Design review of the part built by this model. Coordinates are the model's own, in mm. Face numbers are marked on the shaded views. A direction names the side the tool comes from. Round coordinates to 2 decimals unless told otherwise and drop trailing zeros. Write each loop counter-clockwise with the first axis right and the second up, starting at its lowest first coordinate (ties: lowest second). Pieces come first, ordered by that corner, then holes. Notation, with made-up numbers: M 3,49.25 L 46,49.25 A36 ccw 46,83.25 Z; hole C -37,11.5 d4. An arc over 180 degrees is marked long. Use CSV: the item, a comma, the result in double quotes.
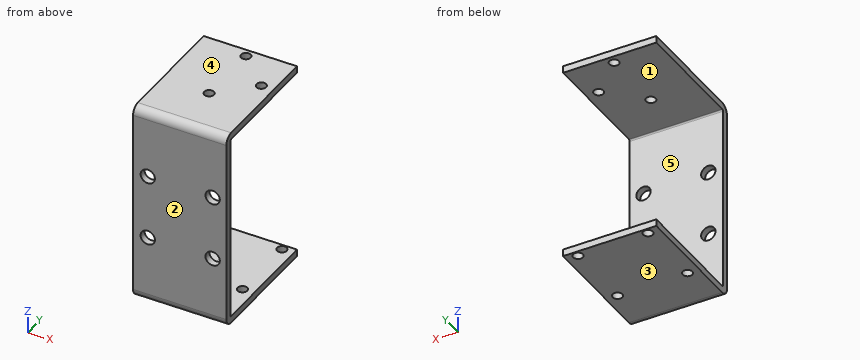
Autodesk Inventor part; units mm, degrees
ref_plane "YZ Plane" through (0, 0, 0) normal (1, 0, 0) x (0, 1, 0)
ref_plane "XZ Plane" through (0, 0, 0) normal (0, 1, 0) x (-1, 0, 0)
ref_plane "XY Plane" through (0, 0, 0) normal (0, 0, 1) x (1, 0, 0)
sketch "Sketch1" plane through (0, 0, 0) normal (0, 1, 0) x (-1, 0, 0)
  line L0 (10.17, 20.25) -> (-9.97, 20.25)
  line L1 (-9.97, 20.25) -> (-9.97, -20.25)
  line L2 (-9.97, -20.25) -> (10.17, -20.25)
  line L3 (10.17, -20.25) -> (10.17, 20.25)
  point P0 (0, 0)
  dimension "d0" = 40.5
  dimension "d1" = 20.14
  dimension "d2" = 10.17
  dimension "d3" = 20.25
extrude "Plate1" add sketch "Sketch1" along normal blind 1.5
sketch "Sketch2" plane through (9.97, 0, 21.75) normal (0, 0, -1) x (-1, 0, 0)
  line L0 (20.14, 0) -> (0, 0)
  line L1 (0, 0) -> (0, 26.9)
  line L2 (0, 26.9) -> (20.14, 26.9)
  line L3 (20.14, 26.9) -> (20.14, 0)
edge flange "Flange1" height 26.9 angle 90 thickness 1.5 bend radius 0.31 thickness toward (0, 0, -1) relief tear relief width 1.5 relief depth 0.75 corner gap 0.31 corner form 0 edges at (-0.1, 1.5, 20.25) (-0.1, 1.5, -20.25) wall of the first edge with corners at (-10.17, 0, 21.75) (9.97, 0, 21.75) (9.97, 26.9, 21.75) (-10.17, 26.9, 21.75)
bend "Bend1"
corner "Corner1"
sketch "Sketch3" plane through (-10.17, 26.9, 21.75) normal (0, 0, 1) x (1, 0, 0)
  circle A0 centre (10.16, -1.83) radius 0.7835
  circle A1 centre (10.16, -15.83) radius 0.7835
  circle A2 centre (17.46, -8.83) radius 0.7835
  point P0 (10.17, -26.9)
hole "Hole1" at (-0.01, 25.07, 21.75) at (7.29, 18.07, 21.75) at (-0.01, 11.07, 21.75) direction (0, 0, -1) diameter 2.1 depth 1.5
sketch "Sketch4" plane through (9.97, 26.9, -21.75) normal (0, 0, -1) x (-1, 0, 0)
  circle A0 centre (2.5, -16.355) radius 0.7835
  circle A1 centre (17.6, -16.355) radius 0.7835
  circle A2 centre (17.6, -1.305) radius 0.7835
  circle A3 centre (2.5, -1.305) radius 0.7835
  point P0 (9.97, -26.9)
hole "Hole2" at (-7.63, 25.595, -21.75) at (-7.63, 10.545, -21.75) at (7.47, 10.545, -21.75) at (7.47, 25.595, -21.75) direction (0, 0, 1) diameter 2.1 depth 1.5
sketch "Sketch5" plane through (0, 0, 0) normal (0, -1, 0) x (1, 0, 0)
  circle A0 centre (-7, 7.0007) radius 1.55
  circle A1 centre (7, 7) radius 1.55
  circle A2 centre (7, -7) radius 1.55
  circle A3 centre (-7, -7) radius 1.55
  point P0 (0, 0)
  dimension "d29" = 3.1
  dimension "d30" = 7
  dimension "d31" = 9.9
  dimension "d32" = 3.1
  dimension "d33" = 7
  dimension "d34" = 7
  dimension "d35" = 3.1
  dimension "d36" = 7
  dimension "d37" = 7
  dimension "d38" = 3.1
  dimension "d39" = 7
  dimension "d40" = 7
extrude "Cut1" cut sketch "Sketch5" against normal blind 1.5
equation "\"d20\" = Thickness"
equation "\"d27\" = Thickness"
equation "\"d41\" = Thickness"
equation "\"d4\" = Thickness"
equation "\"d5\" = BendReliefWidth"
equation "\"d6\" = BendReliefDepth"
equation "\"d7\" = MinimumRemnant"
equation "\"d8\" = TransitionRadius"
equation "\"d11\" = BendRadius"
equation "\"d12\" = CornerReliefSize"
equation "\"d13\" = GapSize"
equation "\"d14\" = JacobiRadiusSize"
equation "\"BendReliefWidth\" = Thickness"
equation "\"BendReliefDepth\" = 0.5 * Thickness"
equation "\"CornerReliefSize\" = 4 * Thickness"
equation "\"MinimumRemnant\" = 2 * Thickness"
equation "\"TransitionRadius\" = BendRadius"
equation "\"JacobiRadiusSize\" = BendRadius"
equation "\"GapSize\" = Thickness"
properties part number "axis_25_bottom_frame" material "Aluminum 6061-AHC"
1) Add section D-D on x = -7.63. Give the number of separate pieces and of enclosed holes in the cut face, then the cut area to 3 significant figures.
Answers:
separate pieces,"5"
enclosed holes,"0"
area,"125 mm²"
2) Add section A-A on y = 10.5. Write out the cut boundary in (x, z), then the cut area to 3 significant figures.
Answers:
outline,"M -10.17,-21.75 L -8.68,-21.75 L -8.68,-20.25 L -10.17,-20.25 Z; M -10.17,20.25 L -0.89,20.25 L -0.89,21.75 L -10.17,21.75 Z; M -6.58,-21.75 L 6.42,-21.75 L 6.42,-20.25 L -6.58,-20.25 Z; M 0.87,20.25 L 9.97,20.25 L 9.97,21.75 L 0.87,21.75 Z; M 8.52,-21.75 L 9.97,-21.75 L 9.97,-20.25 L 8.52,-20.25 Z"
area,"51.5 mm²"
3) Add section C-C on x = -4.5. Write out the cut boundary in (y, z), then the cut area to 3 significant figures.
Answers:
outline,"M 0,-19.94 A1.81 ccw 1.81,-21.75 L 26.9,-21.75 L 26.9,-20.25 L 1.81,-20.25 A0.31 cw 1.5,-19.94 L 1.5,19.94 A0.31 cw 1.81,20.25 L 26.9,20.25 L 26.9,21.75 L 1.81,21.75 A1.81 ccw 0,19.94 Z"
area,"140 mm²"
4) For pin 1 Ø6 at (x, z) = (-2.5, 8) entering from +Y; pin 2 Ø1.3 at (x, y) = (-0.01, 25.07) entering from +Z; pin 3 Ø1.3 at (x, y) = (7.47, 25.595) entering from -Z; pin 4 Ø8 at (y, z) = (6, -8.5) entering from -X, all flat-tipped, find the tip position at first contact; note any pin that passes through.
Answers:
pin 1,"y = 1.5"
pin 2,"z = -20.25"
pin 3,"z = 20.25"
pin 4,"through"
5) The part is to be moulded in two halves that separate along Z. For the marked faces 3, 4 and 5, say which applies: released by +Z, released by -Z, zero draft, split by the parting line, or undercut.
Answers:
face 3,"released by -Z"
face 4,"released by +Z"
face 5,"undercut"
6) Add section B-B on z = -7.5. Write out the cut boundary in (x, y), then the cut area to 3 significant figures.
Answers:
outline,"M -10.17,0 L -8.47,0 L -8.47,1.5 L -10.17,1.5 Z; M -5.53,0 L 5.53,0 L 5.53,1.5 L -5.53,1.5 Z; M 8.47,0 L 9.97,0 L 9.97,1.5 L 8.47,1.5 Z"
area,"21.4 mm²"
7) Machinability: for the marked faces 1 and 2, which of the approach directions +Z, -Z, +X, -X, +Y, -Y give a long, thin tool a straight path to every point of the face, cutting with its end or side? Answer none if there is none.
Answers:
face 1,"+X, -X, +Y"
face 2,"+Z, -Z, +X, -X, -Y"
8) Wall thickness on line 1 along Z through (x, y) = (1, 23.75); line 2 along Y through (x, z) = (-0.01, 21.2); line 3 along Y through (x, z) = (-0.01, 20.7): over which ranges is each line inside the solid? List them lowest first. Write a range as [from, to].
Answers:
line 1,"[-21.75, -20.25], [20.25, 21.75]"
line 2,"[0.51, 10.02], [12.12, 24.02], [26.12, 26.9]"
line 3,"[0.17, 10.02], [12.12, 24.02], [26.12, 26.9]"
